Check sheet for the drawn part. Datum: minimum x, y, z corner. Units: mm. A direction names the side the tool comes from. Coordinates: 2 decimals unless noted, no trailing zeros. Write each loop counter-clockwise with the first axis right and the second up, starting at its lowest first coordinate (ties: lowest second). Pieces come first, ordered by that corner, then holes. Notation, with made-up numbers: (69, 61) -> (104, 61) arc R11 ccw to (104, 72) -> close; hole circle Ø1 at (-24.5, 86). An arc over 180 degrees is marked (long way). Answer in a Markdown table with one row per item. Add a question column.
1. Scan lines: L1, parallel to X at y = 4, z = 12.75 (1 decimal); L2, parallel to Z at x = 7, y = 21.5; L3, parallel to Y at x = 30, z = 6 (1 decimal). Record each from-to range of solid material in increasing order. Write a range as from..to.
2. Cross-section at C-C on y = 25. Record the cut outline in (x, z).
3. Cross-section at A-A on z = 10. Give the number of separate pieces and of enclosed holes in the cut face, and give its area (3 significant figures).
4. Depth check by flat-ended pin: P1, Ø6.5, axis at x = 3.5, z = 6.5, coming from the +Y side; P2, Ø7, axis at y = 37.5, z = 13.5, coming from the -X side; P3, Ø1, axis at y = 34, z = 4.5, coming from the +X side. Enter the tip coordinate at first touch or a pass-through.
5. Set-up check for the marked faces 1, 2 and 3: record each of +Z, -Z, +X, -X, +Y, -Y from which the full face is reachable in a straight line by a thin tool's end or side.
6. Mould release check, pull along Y, two halves, no side actions. Record for the marked faces 4, 5, 6 and 7: pulls with the +Y half, pulls with the -Y half, needs draft (parallel to the pull), parting line crosses it, or undercut.
7. Cross-section at D-D on z = 5. Record the cut outline in (x, y) (1 decimal), and give its area (3 significant figures).
8. Cross-section at B-B on x = 7. Record the cut outline in (y, z).
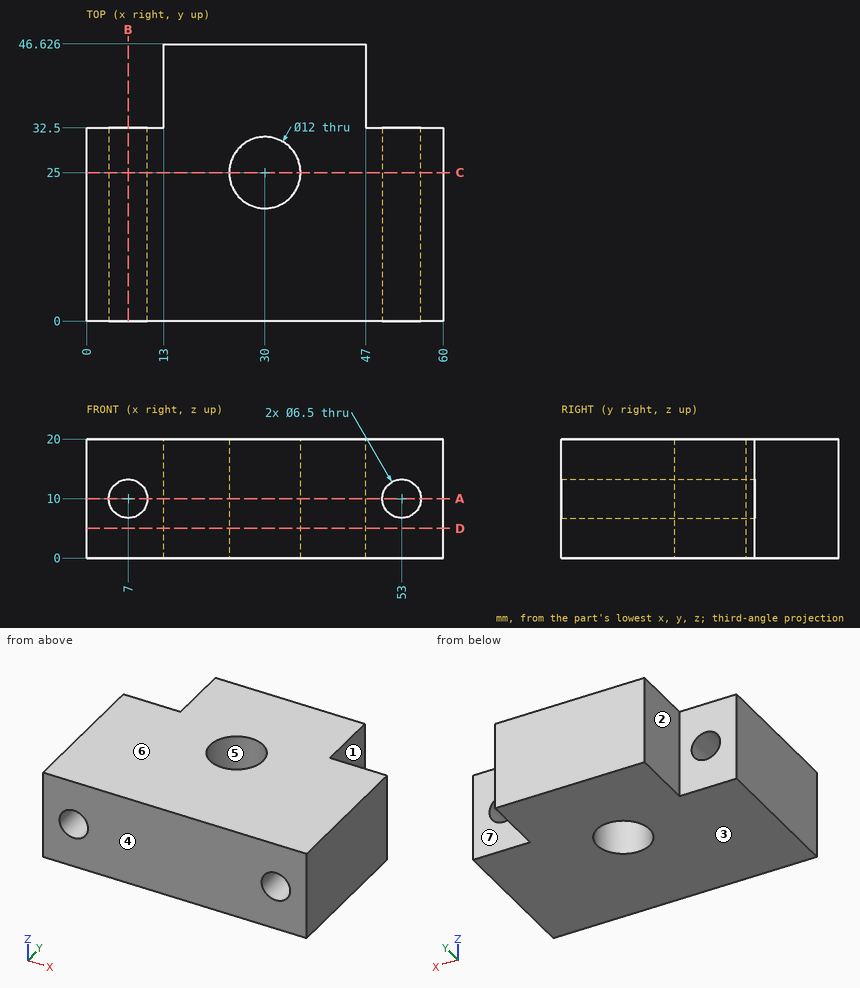
Results found:
| question | item | result |
|---|---|---|
| 1 | L1 | x = 0..5.3, 8.7..51.3, 54.7..60 |
| 1 | L2 | z = 0..6.75, 13.25..20 |
| 1 | L3 | y = 0..19, 31..46.6 |
| 2 | outline | (0, 0) -> (24, 0) -> (24, 20) -> (0, 20) -> close; (36, 0) -> (60, 0) -> (60, 20) -> (36, 20) -> close; hole circle Ø6.5 at (7, 10); hole circle Ø6.5 at (53, 10) |
| 3 | separate pieces | 3 |
| 3 | enclosed holes | 1 |
| 3 | area | 1,890 mm^2 |
| 4 | P1 | stops at y = 32.5 |
| 4 | P2 | stops at x = 13 |
| 4 | P3 | stops at x = 47 |
| 5 | face 1 | +Z, -Z, +X, +Y |
| 5 | face 2 | +Z, -Z, -X, +Y |
| 5 | face 3 | -Z, +X, -X, +Y, -Y |
| 6 | face 4 | pulls with the -Y half |
| 6 | face 5 | undercut |
| 6 | face 6 | needs draft |
| 6 | face 7 | pulls with the +Y half |
| 7 | outline | (0, 0) -> (60, 0) -> (60, 32.5) -> (47, 32.5) -> (47, 46.6) -> (13, 46.6) -> (13, 32.5) -> (0, 32.5) -> close; hole circle Ø12 at (30, 25) |
| 7 | area | 2,320 mm^2 |
| 8 | outline | (0, 0) -> (32.5, 0) -> (32.5, 6.75) -> (0, 6.75) -> close; (0, 13.25) -> (32.5, 13.25) -> (32.5, 20) -> (0, 20) -> close |
